Work out the finished part from the listing and answer in its coordinate system (mm). A direction names the side the tool comes from. Round coordinates to 2 decimals unless told otherwise and drop trailing zeros. Loops run counter-clockwise (first coordinate to the right, second up) from the corner with the lowest first, then second, coordinate; pieces in that order, holes last. Notation, with made-up numbers: (37.5, -1) -> (44.5, -1) arc R32 cw to (44.5, 30) -> close; hole circle Ø4 at (-19.75, -12). An arc over 180 degrees is marked (long way). Write item = value, one per line. Start each with the question number.
```python
from build123d import *

# Parameters (mm, degrees)
F1_DEPTH = 10
F3_DEPTH = 5
F4_R     = 5
F5_W     = 13
F5_H     = 5.2037292719
F6_DEPTH = 5
F7_R     = 4.99999


# Not quite as in the source:
# - a fillet or chamfer is up to 0.001 mm smaller than in the source, because OpenCascade refuses the exact size


with BuildPart() as f1:
    # F0 (on Front) → F1 (new body)
    with BuildSketch(Plane.XZ):
        Polygon((-10.9377613165, 42.7635207549), (-15.9377613165, 42.7635207549), (-15.9377613165, -6.2364792451), (7.0622386835, -6.2364792451), (7.0622386835, 42.7635207549), (2.0622386835, 42.7635207549), (2.0622386835, 21.7635207549), (-10.9377613165, 21.7635207549), align=None)
    extrude(amount=F1_DEPTH)

    # F2 (on face) → F3 (join)
    with BuildSketch(Plane(origin=(0, 0, -6.2364792451), x_dir=(1, 0, 0), z_dir=(0, 0, -1))):
        with BuildLine():
            Line((7.0622386835, 10), (7.0622386835, 0))
            ThreePointArc((7.0622386835, 0), (-4.4377613165, 25.9396283258), (-15.9377613165, 0))
            Line((-15.9377613165, 0), (-15.9377613165, 10))
            Line((-15.9377613165, 10), (7.0622386835, 10))
        make_face()
    extrude(amount=-F3_DEPTH)

    # F4
    f4_edges = [f1.edges().sort_by_distance(p)[0] for p in [
        (-15.937761, -10, 20.763521),
        (7.062239, -10, 20.763521),
    ]]
    fillet(f4_edges, radius=F4_R)

    # F5 (on face) → F6 (join)
    with BuildSketch(Plane.XY.offset(-1.2364792451)):
        with Locations((-4.4377613165, -12.6018646359)):
            Rectangle(F5_W, F5_H)
    extrude(amount=F6_DEPTH)

    # F7 (radius 5 in the source; OpenCascade refuses exactly that, so slightly less here)
    f7_edges = [f1.edges().sort_by_distance(p)[0] for p in [
        (-4.437761, -15.203729, 3.763521),
    ]]
    fillet(f7_edges, radius=F7_R)


solid = f1.part
```
Item 1: Find the intervals of material crossed by line 1 along X through (y, z) = (-3, 36); line 2 along Z through (x, y) = (-17.5, -2.75); line 3 along X through (y, z) = (-2.5, 3), in increasing order. Write a range as [from, to].
Item 2: Section C-C (y = -6.75) is taken. Determine the outline of the cut face in (x, z).
Item 3: The mould has two halves that part along X. Classify faces 1 (the flat face through (2.062, -5, 32)), 2 (the flat face through (7.062, -2, 20)), 3 (the flat face through (-5, -16, -1.236)): pulls with the +X half, pulls with the -X half, needs draft (parallel to the pull), parting line crosses it, or undercut.
Item 4: A tool of negligible diameter and unlimited length cuts with its end or side. For faces 4 (the flat face through (-15.938, -2, 21)), 5 (the flat face through (2.062, -12, 1)), 6 (the flat face through (-4, -5, 21.764)), 7 (the cylindrical face through (-14.51, -8.5, 20.46)), from which of +Z, -Z, +X, -X, +Y, -Y can it reach the whole face along a straight path? Write none if from no direction.
Item 5: Section A-A (z = 30.5) is taken. Determine the outline of the cut face in (x, y).
Item 6: Section B-B (z = 8.5) is taken. Determine the outline of the cut face in (x, y), then the cut area to 3 significant figures.
Item 7: Flat-ended cylindrical pins translate along their axes: pin 1 (11 mm diameter, centred on x = -4.5, y = -3.5, fed in from +Z); pin 2 (5 mm diameter, centred on y = -4.5, z = 34, fed in from -X); pin 3 (6 mm diameter, centred on x = 1, y = -21.5, fed in from +Z). Find the tip coordinate at first contact, or state that the pin passes through.
Worked answers:
q1.line_1 = [-15.94, -10.94], [2.06, 7.06]
q1.line_2 = [-6.24, -1.24]
q1.line_3 = [-15.94, 7.06]
q2.outline = (-19.52, -6.24) -> (10.64, -6.24) -> (10.64, -1.24) -> (6.75, -1.24) -> (6.75, 42.76) -> (2.06, 42.76) -> (2.06, 21.76) -> (-10.94, 21.76) -> (-10.94, 42.76) -> (-15.62, 42.76) -> (-15.62, -1.24) -> (-19.52, -1.24) -> close
q3.face_1 = undercut
q3.face_2 = pulls with the +X half
q3.face_3 = needs draft
q4.face_4 = +Z, -X, +Y, -Y
q4.face_5 = +Z, +X, -Y
q4.face_6 = +Z, +Y, -Y
q4.face_7 = +Z, -X, -Y
q5.outline = (-15.94, -5) arc R5 ccw to (-10.94, -10) -> (-10.94, 0) -> (-15.94, 0) -> close; (2.06, -10) arc R5 ccw to (7.06, -5) -> (7.06, 0) -> (2.06, 0) -> close
q6.outline = (-15.94, -5) arc R5 ccw to (-10.94, -10) -> (2.06, -10) arc R5 ccw to (7.06, -5) -> (7.06, 0) -> (-15.94, 0) -> close
q6.area = 219 mm2
q7.pin_1 = 21.76
q7.pin_2 = -15.94
q7.pin_3 = -1.24
